Check sheet for the modelled part. Datum: model origin and axes. Units: mm. A direction names the side the tool comes from. Give positions to 0.01 mm unless a question says otherwise; leave off trailing zeros. Loops run counter-clockwise (first coordinate to the right, second up) from the corner with the lowest first, then second, coordinate; pieces in that order, holes last. Notation, with made-up numbers: (22, 37.25) - (69, 37.25) arc R30 cw to (69, 62.25) - close; hole circle Ø10 at (33.25, 74.25). An arc over 180 degrees is marked (long way). Use one line per item in the form item = value.
from build123d import *

# Parameters (mm, degrees)
SALIENTE_EXTRUIR1_DEPTH = 14.8
CORTAR_EXTRUIR1_DEPTH   = 10.05
CROQUIS2_R              = 1.6
CORTAR_EXTRUIR2_DEPTH   = 5


with BuildPart() as part:
    # Croquis1 → Saliente-Extruir1 (new body)
    with BuildSketch(Plane(origin=(0, 0, 0), x_dir=(1, 0, 0), z_dir=(0, 1, 0))):
        Polygon((1.977424672, -3.425), (3.954849344, 0), (1.977424672, 3.425), (-1.977424672, 3.425), (-3.954849344, 0), (-1.977424672, -3.425), align=None)
    extrude(amount=SALIENTE_EXTRUIR1_DEPTH)

    # Croquis1_3 → Cortar-Extruir1 (cut)
    with BuildSketch(Plane(origin=(0, 0, 0), x_dir=(1, 0, 0), z_dir=(0, 1, 0))):
        Polygon((-2.800148806, 0), (-1.400074403, -2.425), (1.400074403, -2.425), (2.800148806, 0), (1.400074403, 2.425), (-1.400074403, 2.425), align=None)
    extrude(amount=CORTAR_EXTRUIR1_DEPTH, mode=Mode.SUBTRACT)

    # Croquis2 → Cortar-Extruir2 (cut)
    with BuildSketch(Plane(origin=(0, 14.8, 0), x_dir=(1, 0, 0), z_dir=(0, 1, 0))):
        with Locations(Location((0, 0, 0), (0, 0, 270))):
            Circle(CROQUIS2_R)
    extrude(amount=-CORTAR_EXTRUIR2_DEPTH, mode=Mode.SUBTRACT)


solid = part.part
Item 1: Gauge pin test, flat end, axial feed: P1, Ø3, axis at x = 0, z = 0, coming from the +Y side. Record the tip position at first contact, or that the pin passes through.
Answer block:
P1 = through
Item 2: Thickness scan on L1, parallel to Z at x = 0.25, y = 8.75 (3 decimals); L2, parallel to X at y = 5.5, z = -0.5; L3, parallel to X at y = 7.25, z = -2. Record the ranges inside material, lowest first.
Answer block:
L1 = -3.425 to -2.425, 2.425 to 3.425
L2 = -3.67 to -2.51, 2.51 to 3.67
L3 = -2.8 to -1.65, 1.65 to 2.8
Item 3: Section check D-D on z = -2. Record the boundary of the cut face in (x, y).
Answer block:
outline = (-2.8, 0) - (-1.65, 0) - (-1.65, 10.05) - (1.65, 10.05) - (1.65, 0) - (2.8, 0) - (2.8, 14.8) - (-2.8, 14.8) - close
Item 4: Section check B-B on x = 0. Record the boundary of the cut face in (y, z) (3 decimals), then the cut area to 3 significant figures.
Answer block:
outline = (0, -3.425) - (14.8, -3.425) - (14.8, -1.6) - (10.05, -1.6) - (10.05, -2.425) - (0, -2.425) - close; (0, 2.425) - (10.05, 2.425) - (10.05, 1.6) - (14.8, 1.6) - (14.8, 3.425) - (0, 3.425) - close
area = 37.4 mm2
Item 5: Access from +Z, -Z, +X, -X, +Y, -Y to the whole of each face (thin tool, end or side, straight path). Record for faces 4 (the face through (-2.09, 4.95, -1.23)), 5 (the face through (-0.97, 12.46, -1.27)).
Answer block:
face_4 = -Y
face_5 = +Y, -Y
Item 6: Section check A-A on y = 6.75. Record the boundary of the cut face in (x, z) (3 decimals).
Answer block:
outline = (-3.955, 0) - (-1.977, -3.425) - (1.977, -3.425) - (3.955, 0) - (1.977, 3.425) - (-1.977, 3.425) - close; hole (-2.8, 0) - (-1.4, -2.425) - (1.4, -2.425) - (2.8, 0) - (1.4, 2.425) - (-1.4, 2.425) - close
Item 7: Section check C-C on z = -1.25. Record the boundary of the cut face in (x, y).
Answer block:
outline = (-3.23, 0) - (-2.08, 0) - (-2.08, 10.05) - (-1, 10.05) - (-1, 14.8) - (-3.23, 14.8) - close; (1, 10.05) - (2.08, 10.05) - (2.08, 0) - (3.23, 0) - (3.23, 14.8) - (1, 14.8) - close
Item 8: Mould release check, pull along X, two halves, no side actions. Record for faces 1 (the face through (-2.11, 4.955, 1.196)), 2 (the face through (2.98, 7.3, -1.69)), 3 (the face through (0, 7, 3.425)): released by +X, released by -X, zero draft, split by the parting line, or undercut.
Answer block:
face_1 = undercut
face_2 = released by +X
face_3 = zero draft
